from build123d import *

# Parameters (mm, degrees)
F0_W     = 250
F0_H     = 75
F1_DEPTH = 25
F2_R     = 5
F4_D     = 29
F5_D     = 29
F6_D     = 29


with BuildPart() as f1:
    # F0 (on Top) → F1 (new body, symmetric)
    with BuildSketch(Plane.XY):
        with Locations((-125, 37.5)):
            Rectangle(F0_W, F0_H)
    extrude(amount=F1_DEPTH, both=True)

    # F2
    f2_edges = [f1.edges().sort_by_distance(p)[0] for p in [
        (0, 37.5, 25),
        (0, 0, 0),
        (0, 37.5, -25),
        (0, 75, 0),
        (-125, 0, -25),
        (-125, 0, 25),
        (-250, 0, 0),
        (-250, 37.5, 25),
        (-250, 75, 0),
        (-250, 37.5, -25),
        (-125, 75, -25),
        (-125, 75, 25),
    ]]
    fillet(f2_edges, radius=F2_R)

    # F4 (through all)
    with Locations(Plane.XY.offset(25)):
        with Locations((-128.644977, 40.611042)):
            Hole(F4_D / 2)

    # F5 (through all)
    with Locations(Plane.XY.offset(25)):
        with Locations((-39.162696, 43.24426)):
            Hole(F5_D / 2)

    # F6 (through all)
    with Locations(Plane.XY.offset(25)):
        with Locations((-218.127259, 37.977825)):
            Hole(F6_D / 2)


solid = f1.part
Design review of the part built by this model. Coordinates are the model's own, in mm. Round coordinates to 2 decimals unless told otherwise and drop trailing zeros. Write each loop counter-clockwise with the first axis right and the second up, starting at its lowest first coordinate (ties: lowest second). Pieces come first, ordered by that corner, then holes.
Item 1: Wall thickness on L1, parallel to X at y = 25, z = 15; L2, parallel to X at y = 26, z = -8.5; L3, parallel to Y at x = -222, z = 20.5: over which ranges is each line inside the solid? List them lowest first.
Item 2: Consider section C-C on z = 10. Give the boundary of the cut face in (x, y), and give its area (3 significant figures).
Item 3: For pin 1 Ø10 at (x, y) = (-34, 43) entering from +Z, flat-tipped, find the tip position at first contact; note if it passes through.
Item 4: Consider section D-D on x = -131.5. Give the boundary of the cut face in (y, z), and give its area (3 significant figures).
Item 5: Consider section A-A on y = 32.5. Give the boundary of the cut face in (x, z).
Item 6: Consider section B-B on x = -227.5. Give the boundary of the cut face in (y, z), and give its area (3 significant figures).
Item 7: Draft analysis for pull direction Y (two halves, no side actions). For faces 1 (the flat face through (-127, 0, 0)), 2 (the cylindrical face through (-2, 38, 24)), 3 (the cylindrical face through (-231.96, 42.33, -0.35)), state which applies: released by +Y, released by -Y, zero draft, split by the parting line, or undercut.
Check values:
1. L1: x = -250 to -224.59, -211.66 to 0
1. L2: x = -250 to -226.3, -209.96 to 0
1. L3: y = 0.03 to 24, 51.95 to 74.97
2. outline: (-250, 5) arc R5 ccw to (-245, 0) - (-5, 0) arc R5 ccw to (0, 5) - (0, 70) arc R5 ccw to (-5, 75) - (-245, 75) arc R5 ccw to (-250, 70) - close; hole circle Ø29 at (-218.13, 37.98); hole circle Ø29 at (-128.64, 40.61); hole circle Ø29 at (-39.16, 43.24)
2. area: 16,700 mm2
3. pin 1: passes through
4. outline: (0, -20) arc R5 ccw to (5, -25) - (26.39, -25) - (26.39, 25) - (5, 25) arc R5 ccw to (0, 20) - close; (54.83, -25) - (70, -25) arc R5 ccw to (75, -20) - (75, 20) arc R5 ccw to (70, 25) - (54.83, 25) - close
4. area: 2,310 mm2
5. outline: (-250, -20) arc R5 ccw to (-245, -25) - (-231.55, -25) - (-231.55, 25) - (-245, 25) arc R5 ccw to (-250, 20) - close; (-204.7, -25) - (-140.66, -25) - (-140.66, 25) - (-204.7, 25) - close; (-116.63, -25) - (-48.9, -25) - (-48.9, 25) - (-116.63, 25) - close; (-29.43, -25) - (-5, -25) arc R5 ccw to (0, -20) - (0, 20) arc R5 ccw to (-5, 25) - (-29.43, 25) - close
6. outline: (0, -20) arc R5 ccw to (5, -25) - (26.91, -25) - (26.91, 25) - (5, 25) arc R5 ccw to (0, 20) - close; (49.04, -25) - (70, -25) arc R5 ccw to (75, -20) - (75, 20) arc R5 ccw to (70, 25) - (49.04, 25) - close
6. area: 2,620 mm2
7. face 1: released by -Y
7. face 2: zero draft
7. face 3: undercut
